For this review, take the finished solid that the model builds, in its own axes (mm). Face numbers are marked on the shaded views. A direction names the side the tool comes from. Round coordinates to 2 decimals unless told otherwise and drop trailing zeros. Write each loop counter-clockwise with the first axis right and the second up, starting at its lowest first coordinate (ties: lowest second). Pieces come first, ordered by that corner, then holes. Notation, with made-up numbers: (-3.75, 49) -> (24.25, 49) arc R8 cw to (24.25, 60) -> close; hole circle Ø2 at (39, 5). An arc over 180 degrees is marked (long way). Answer as CSV lines item,"result". Start each with the question number.
Item 1: Machinability: for the marked faces 1 and 2, which of the approach directions +Z, -Z, +X, -X, +Y, -Y give a long, thin tool a straight path to every point of the face, cutting with its end or side? Answer none if there is none.
Item 2: Wall thickness on probe 1 along X at (y, z) = (61.5, 4.5); probe 2 along X at (y, z) = (77, -4.5); probe 3 along Y at (x, z) = (-1, -2.5): over which ranges is each line inside the solid? List them lowest first. Write a range as from..to.
Item 3: For pin 1 Ø6 at (x, z) = (36.5, 2) entering from +Y; pin 2 Ø3 at (x, z) = (24.5, 3.5) entering from +Y; pin 3 Ø3 at (x, z) = (6.5, 0.5) entering from +Y, all flat-tipped, find the tip position at first contact; note any pin that passes through.
Item 4: Take a section at C-C on x = 27.5. Give the boundary of the cut face in (y, z), then the cut area to 3 significant figures.
Item 5: Take a section at B-B on y = 62.5. Give the boundary of the cut face in (x, z), then the cut area to 3 significant figures.
Item 6: Mouldability with a two-part tool opening along X and no side actions: class the marked faces 3, 4 and 5 as +X half, -X half, draft (parallel to the pull), parting line (faces both ways), or undercut.
Item 7: Take a section at A-A on z = -3.25. Give the boundary of the cut face in (x, y), then the cut area to 3 significant figures.
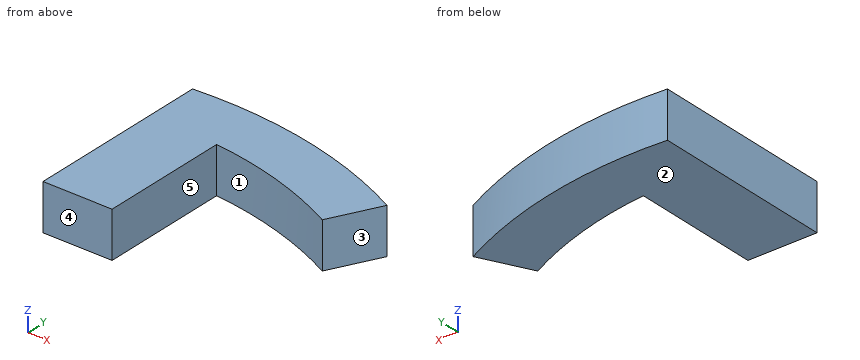
```python
from build123d import *

# Parameters (mm, degrees)
BOSS_EXTRUDE1_DEPTH = 5


with BuildPart() as part:
    # Sketch1 → Boss-Extrude1 (new body, symmetric)
    with BuildSketch(Plane.XY):
        with BuildLine():
            Line((37.953605778, 74.488145422), (43.401491775, 85.180223712))
            ThreePointArc((43.401491775, 85.180223712), (18.896814133, 93.713768549), (-7, 95.343379424))
            Line((-7, 95.343379424), (-7, 55))
            Line((-7, 55), (0, 55))
            Line((0, 55), (8, 55))
            Line((8, 55), (8, 83.216344548))
            ThreePointArc((8, 83.216344548), (23.387578669, 80.261953403), (37.953605778, 74.488145422))
        make_face()
    extrude(amount=BOSS_EXTRUDE1_DEPTH, both=True)


solid = part.part
```
Output values:
1,face 1,"+Z, -Z, -Y"
1,face 2,"-Z, +X, -X, +Y, -Y"
2,probe 1,"x = -7..8"
2,probe 2,"x = -7..8, 32.56..39.23"
2,probe 3,"y = 55..95.59"
3,pin 1,"stops at y = 89.54"
3,pin 2,"stops at y = 92.79"
3,pin 3,"stops at y = 95.47"
4,outline,"(78.95, -5) -> (91.56, -5) -> (91.56, 5) -> (78.95, 5) -> close"
4,area,"126 mm^2"
5,outline,"(-7, -5) -> (8, -5) -> (8, 5) -> (-7, 5) -> close"
5,area,"150 mm^2"
6,face 3,"+X half"
6,face 4,"draft"
6,face 5,"undercut"
7,outline,"(-7, 55) -> (8, 55) -> (8, 83.22) arc R83.6 cw to (37.95, 74.49) -> (43.4, 85.18) arc R95.6 ccw to (-7, 95.34) -> close"
7,area,"1,020 mm^2"
